Source: CAD feature listing. Evaluate the final solid. Frame: model axes, mm. Give positions to 0.01 mm unless a question says otherwise; leave off trailing zeros. Loops run counter-clockwise (first coordinate to the right, second up) from the corner with the lowest first, then second, coordinate; pieces in that order, holes last. Notation, with made-up numbers: (-19, 86.5) -> (13, 86.5) arc R22 cw to (13, 110.5) -> close; hole circle Ø9 at (4, -25). An arc over 180 degrees is marked (long way). Return JSON: item names as keys, results as strings. Group by question number.
(1) Cut plane A-A on x = -19. Return loops of the section in (y, z), then the cut area to 3 significant figures.
(2) Cut plane B-B on z = 5. Give the number of separate pieces and of enclosed holes in the cut face, then the cut area to 3 significant figures.
(3) Ray query, line 1 (Y direction, x = 0, z = 6.65); line 2 (Z direction, x = -23.5, y = -26); line 3 (Y direction, x = 21.5, z = 5.5). Return the intervals inside material, ascending. Write a range as from..to.
(4) Pin query (flat end, axial travel): pin 1 (2 mm diameter, centred on x = -8.5, y = -5, fed in from +Z) (3 decimals); pin 2 (19 mm diameter, centred on x = -1, y = 11.5, fed in from +Z); pin 3 (1.6 mm diameter, centred on x = 10, z = 4, fed in from +Y); pin 4 (4 mm diameter, centred on x = -9, y = -26.5, fed in from -Z). Return the tip coordinate at first contact, or that it passes through.
```python
from build123d import *

# Parameters (mm, degrees)
F3_DEPTH = 3.175


with BuildPart() as f1:
    # F0 (on Front) → F1 (revolve)
    with BuildSketch(Plane.XZ):
        Polygon((-44.60875, 7.366), (-46.99, 7.366), (-46.99, 0), (0, 0), (0, 6.35), (-44.60875, 6.35), align=None)
    revolve(axis=Axis((0, 0, 3.175), (0, 0, -1)))

    # F2 (on face) → F3 (cut)
    with BuildSketch(Plane.XY.offset(6.35)):
        Polygon((-13.136034, 38.912354), (-13.105828, 3.757066), (-11.859001, 3.771245), (-10.660359, 3.537526), (-9.526933, 3.091542), (-8.475764, 2.468926), (-7.523901, 1.705309), (-6.688365, 0.836315), (-5.434484, -1.075276), (-4.651632, -3.288853), (-4.293584, -5.777134), (-4.324106, -7.01164), (-4.521094, -8.179643), (-4.904661, -9.236092), (-5.494886, -10.135925), (-6.268279, -10.791905), (-7.162464, -11.166064), (-8.139243, -11.287278), (-9.160387, -11.184392), (-10.187706, -10.886271), (-11.182993, -10.421768), (-12.924614, -9.109049), (-14.077223, -10.739327), (-15.044289, -12.482277), (-15.832252, -14.317493), (-16.447562, -16.224576), (-16.896672, -18.183107), (-17.186041, -20.17271), (-17.311352, -24.163445), (-16.875112, -28.033535), (-15.92893, -31.619757), (-14.524421, -34.758876), (-13.666418, -36.109751), (-12.713203, -37.287646), (-12.806471, -34.975058), (-12.698982, -32.758747), (-12.410626, -30.64813), (-11.961338, -28.652615), (-11.371018, -26.781629), (-10.65961, -25.04458), (-8.953136, -22.009984), (-7.001257, -19.624146), (-4.963309, -17.962417), (-3.961857, -17.426638), (-2.998644, -17.100127), (-2.093584, -16.99232), (-1.266589, -17.112616), (-0.547738, -17.414856), (0.049097, -17.837887), (0.894188, -18.994107), (1.303621, -20.476849), (1.312331, -22.181665), (0.955265, -24.004137), (0.267348, -25.839818), (-0.716463, -27.584268), (-1.961242, -29.13307), (0.694919, -27.714731), (3.341536, -26.055124), (5.929156, -24.178162), (8.408294, -22.107803), (10.729487, -19.867958), (12.84326, -17.482574), (14.70014, -14.975573), (16.250653, -12.370882), (5.408085, -12.340676), (6.616165, -10.437943), (17.337931, -10.437943), (18.092985, -8.776826), (7.341023, -8.807032), (8.549104, -6.783486), (18.878235, -6.813692), (20.078154, -2.783312), (20.717557, 0.236366), (21.025033, 3.701278), (20.970354, 5.548097), (20.731948, 7.443102), (20.27624, 9.36524), (19.569635, 11.293491), (18.57855, 13.206803), (17.269421, 15.084145), (15.608653, 16.904463), (13.56266, 18.646717), (15.106564, 16.045076), (16.115819, 13.497777), (16.659601, 11.049964), (16.807072, 8.746751), (16.627389, 6.633274), (16.189703, 4.754655), (15.563201, 3.15604), (14.817037, 1.882544), (13.560792, 0.283274), (12.379845, -0.875078), (11.235587, -1.620599), (10.089418, -1.981339), (8.639236, -2.107231), (6.944323, -1.932942), (6.162442, -1.641123), (5.508173, -1.163719), (5.044462, -0.463882), (4.834245, 0.495234), (4.906693, 1.477767), (5.207401, 2.224786), (5.673899, 2.738488), (6.243748, 3.02109), (6.854487, 3.074787), (7.443656, 2.901786), (7.948806, 2.504294), (8.307488, 1.884528), (8.318795, 3.616362), (8.001849, 5.432468), (7.385926, 7.246082), (6.500356, 8.970472), (5.374426, 10.518863), (4.037456, 11.804512), (2.518732, 12.740654), (0.847564, 13.240535), (1.51767, 11.651856), (1.942676, 10.195223), (2.144573, 8.877468), (2.145376, 7.705464), (1.967064, 6.686042), (1.631632, 5.826053), (1.161079, 5.132351), (0.5774, 4.611786), (-0.097415, 4.271211), (-0.841351, 4.117468), (-1.632439, 4.157409), (-2.448655, 4.397884), (-3.268038, 4.845748), (-4.068565, 5.50784), (-4.828243, 6.391013), (-5.525092, 7.502131), (-6.521002, 9.899941), (-6.928186, 12.120486), (-6.816748, 14.054397), (-6.256802, 15.592293), (-5.830562, 16.178549), (-5.318485, 16.624797), (-4.729337, 16.917354), (-4.07189, 17.042549), (-3.354908, 16.986719), (-2.587142, 16.736182), (-1.777377, 16.277264), (-0.934366, 15.596305), (-1.09684, 16.28627), (-1.439569, 16.97463), (-2.579857, 18.435592), (-4.183413, 20.157332), (-6.078396, 22.317982), (-8.092979, 25.095675), (-10.055332, 28.668541), (-10.963232, 30.808836), (-11.793627, 33.214723), (-12.525052, 35.90847), align=None)
        Polygon((-6.518141, -5.256094), (-6.24994, -3.97469), (-6.509726, -2.714876), (-7.249545, -1.646867), (-8.356745, -0.933242), (-9.662781, -0.682651), (-10.968817, -0.933242), (-12.076028, -1.646867), (-12.815836, -2.714876), (-13.075622, -3.97469), (-12.807422, -5.256094), (-12.076028, -6.302502), (-10.99121, -7.008008), (-9.662781, -7.266718), (-8.334352, -7.008008), (-7.249545, -6.302502), align=None)
    extrude(amount=-F3_DEPTH, mode=Mode.SUBTRACT)


solid = f1.part
```
Answers:
{
 "1": {"outline": "(-42.98, 0) -> (42.98, 0) -> (42.98, 7.37) -> (40.36, 7.37) -> (40.36, 6.35) -> (-40.36, 6.35) -> (-40.36, 7.37) -> (-42.98, 7.37) -> close", "area": "551 mm²"},
 "2": {"separate pieces": "1", "enclosed holes": "2", "area": "5,950 mm²"},
 "3": {"line 1": "-46.99..-44.61, 44.61..46.99", "line 2": "0..6.35", "line 3": "-41.78..41.78"},
 "4": {"pin 1": "z = 3.175", "pin 2": "z = 6.35", "pin 3": "y = 46.08", "pin 4": "z = 0"}
}
